Check sheet for the modelled part. Datum: model origin and axes. Units: mm. Face numbers are marked on the shaded views. Coordinates: 2 decimals unless noted, no trailing zeros. Loops run counter-clockwise (first coordinate to the right, second up) from the corner with the lowest first, then second, coordinate; pieces in that order, holes last.
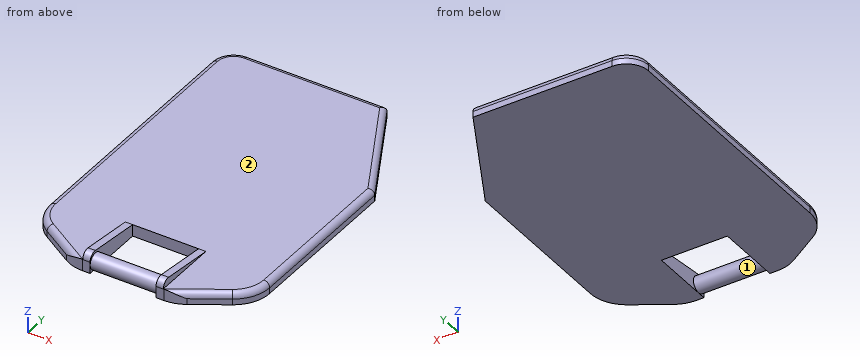
from build123d import *

# Parameters (mm, degrees)
F0_W          = 30
F0_H          = 45
F1_DEPTH      = 1.6
F2_SIZE2      = 8
F2_SIZE       = 5
F2_2_SIZE2    = 8
F2_2_SIZE     = 5
F3_R          = 3
F5_DEPTH      = 1.6
F6_W          = 11
F6_H          = 9
F7_DEPTH      = 2
F8_R          = 5
F10_DEPTH     = 1
F11_T1_DEPTH  = 6.6483183522
F13_DEPTH     = 1
F14_T1_DEPTH  = 6.6483183522
F16_T1_DEPTH  = 34.2287617925
F16_T3_DEPTH  = 24.2287617925
F16_T5_DEPTH  = 21
F16_T7_DEPTH  = 21
F16_T12_DEPTH = 8.6287617925
F16_T17_DEPTH = 8.6287617925
F16_T20_ANGLE = 57.9946167919
F16_T22_ANGLE = 90
F16_T24_ANGLE = 57.9946167919
F15_R         = 1.1066061355
F17_DEPTH     = 9


# Not quite as in the source:
# - a fillet or chamfer that OpenCascade refuses, or shapes differently, is made with other operations: its cross-section is extruded or revolved along the edge and cut away or added


with BuildPart() as f1:
    # F0 (on Top) → F1 (new body)
    with BuildSketch(Plane.XY):
        with Locations((-15, 22.5)):
            Rectangle(F0_W, F0_H)
    extrude(amount=F1_DEPTH)

    # F2
    f2_edges = [f1.edges().sort_by_distance(p)[0] for p in [
        (0, 0, 0.8),
    ]]
    f2_side = f1.faces().sort_by_distance((0, 22.5, 0.8))[0]
    chamfer(f2_edges, length=F2_SIZE, length2=F2_SIZE2, reference=f2_side)

    # F2#2
    f2_2_edges = [f1.edges().sort_by_distance(p)[0] for p in [
        (-30, 0, 0.8),
    ]]
    f2_2_side = f1.faces().sort_by_distance((-30, 22.5, 0.8))[0]
    chamfer(f2_2_edges, length=F2_2_SIZE, length2=F2_2_SIZE2, reference=f2_2_side)

    # F3
    f3_edges = [f1.edges().sort_by_distance(p)[0] for p in [
        (0, 45, 0.8),
        (-30, 45, 0.8),
    ]]
    fillet(f3_edges, radius=F3_R)

    # F4 (on face) → F5 (cut)
    with BuildSketch(Plane(origin=(0, 0, 0), x_dir=(1, 0, 0), z_dir=(0, 0, -1))):
        Polygon((0, -45), (0, -30), (-8, -45), align=None)
    extrude(amount=-F5_DEPTH, mode=Mode.SUBTRACT)

    # F6 (on face) → F7 (cut)
    with BuildSketch(Plane.XY.offset(1.6)):
        with Locations((-15, 4.5)):
            Rectangle(F6_W, F6_H)
    extrude(amount=-F7_DEPTH, mode=Mode.SUBTRACT)

    # F8
    f8_edges = [f1.edges().sort_by_distance(p)[0] for p in [
        (0, 5, 0.8),
        (-8, 0, 0.8),
        (-22, 0, 0.8),
        (-30, 5, 0.8),
    ]]
    fillet(f8_edges, radius=F8_R)

    # F9 (on face) → F10 (join)
    with BuildSketch(Plane(origin=(-9.5, 0, 0), x_dir=(0, -1, 0), z_dir=(-1, 0, 0))):
        Polygon((0, 2.7), (-9, 1.6), (-9, 0), (0, 0), align=None)
    extrude(amount=F10_DEPTH)

    # F11: fillet of radius 1 on 1 edges, made by hand

    # F11_s2 → F11_t1 (cut)
    with BuildSketch(Plane.YZ.offset(-13.3241591761)):
        with BuildLine():
            ThreePointArc((1.12131943, 2.5629498474), (0.3371725073, 2.3191084678), (0, 1.5703363296))
            Line((0, 1.5703363296), (0, 2.7))
            Line((0, 2.7), (1.12131943, 2.5629498474))
        make_face()
    extrude(amount=F11_T1_DEPTH, mode=Mode.SUBTRACT)

    # F12 (on face) → F13 (join)
    with BuildSketch(Plane.YZ.offset(-20.5)):
        Polygon((0, 2.7), (0, 0), (9, 0), (9, 1.6), align=None)
    extrude(amount=F13_DEPTH)

    # F14: fillet of radius 1 on 1 edges, made by hand

    # F14_s2 → F14_t1 (cut)
    with BuildSketch(Plane.YZ.offset(-23.3241591761)):
        with BuildLine():
            ThreePointArc((1.12131943, 2.5629498474), (0.3371725073, 2.3191084678), (0, 1.5703363296))
            Line((0, 1.5703363296), (0, 2.7))
            Line((0, 2.7), (1.12131943, 2.5629498474))
        make_face()
    extrude(amount=F14_T1_DEPTH, mode=Mode.SUBTRACT)

    # F16: fillet of radius 0.8 on 9 edges, made by hand

    # F16_s2 → F16_t1 (cut)
    with BuildSketch(Plane.XZ.offset(-42)):
        with BuildLine():
            ThreePointArc((-30, 0.8), (-29.7656854249, 1.3656854249), (-29.2, 1.6))
            Line((-29.2, 1.6), (-30, 1.6))
            Line((-30, 1.6), (-30, 0.8))
        make_face()
    extrude(amount=F16_T1_DEPTH, mode=Mode.SUBTRACT)

    # F16_s4 → F16_t3 (cut)
    with BuildSketch(Plane.XZ.offset(-32)):
        with BuildLine():
            ThreePointArc((0, 0.8), (-0.2343145751, 1.3656854249), (-0.8, 1.6))
            Line((-0.8, 1.6), (0, 1.6))
            Line((0, 1.6), (0, 0.8))
        make_face()
    extrude(amount=F16_T3_DEPTH, mode=Mode.SUBTRACT)

    # F16_s6 → F16_t5 (cut)
    with BuildSketch(Plane.YZ.offset(-27)):
        with BuildLine():
            ThreePointArc((45, 0.8), (44.7656854249, 1.3656854249), (44.2, 1.6))
            Line((44.2, 1.6), (45, 1.6))
            Line((45, 1.6), (45, 0.8))
        make_face()
    extrude(amount=F16_T5_DEPTH, mode=Mode.SUBTRACT)

    # F16_s8 → F16_t7 (cut)
    with BuildSketch(Plane(origin=(-11.5155709343, 21.5916955017, 0), x_dir=(0, 0, 1), z_dir=(-0.4705882353, 0.8823529412, 0))):
        with BuildLine():
            ThreePointArc((0.8, 14.1176470588), (1.3656854249, 13.8833324838), (1.6, 13.3176470588))
            Line((1.6, 13.3176470588), (1.6, 14.1176470588))
            Line((1.6, 14.1176470588), (0.8, 14.1176470588))
        make_face()
    extrude(amount=F16_T7_DEPTH, mode=Mode.SUBTRACT)


with BuildPart() as f16_tool10:
    # F16_s11 → F16_t12 (new body)
    with BuildSketch(Plane(origin=(-21.4702194191, 13.4188871369, 0), x_dir=(0, 0, 1), z_dir=(0.847998304, -0.52999894, 0))):
        with BuildLine():
            ThreePointArc((0.8, 11.6599766801), (1.3656854249, 11.425662105), (1.6, 10.8599766801))
            Line((1.6, 10.8599766801), (1.6, 11.6599766801))
            Line((1.6, 11.6599766801), (0.8, 11.6599766801))
        make_face()
    extrude(amount=F16_T12_DEPTH)

    split(bisect_by=Plane.YZ.offset(-20.5), keep=Keep.BOTTOM)


with BuildPart() as f1_1:
    add(f1.part)

    # F16_t9: cut F16_tool10
    add(f16_tool10.part, mode=Mode.SUBTRACT)


with BuildPart() as f16_tool15:
    # F16_s16 → F16_t17 (new body)
    with BuildSketch(Plane(origin=(-0.1028142887, -0.0642589305, 0), x_dir=(0, 0, 1), z_dir=(-0.847998304, -0.52999894, 0))):
        with BuildLine():
            ThreePointArc((0.8, 4.23999152), (1.3656854249, 4.4743060951), (1.6, 5.03999152))
            Line((1.6, 5.03999152), (1.6, 4.23999152))
            Line((1.6, 4.23999152), (0.8, 4.23999152))
        make_face()
    extrude(amount=F16_T17_DEPTH)

    split(bisect_by=Plane.YZ.offset(-9.5), keep=Keep.TOP)


with BuildPart() as f1_2:
    add(f1_1.part)

    # F16_t14: cut F16_tool15
    add(f16_tool15.part, mode=Mode.SUBTRACT)

    # F16_s19 → F16_t20 (revolve, cut)
    with BuildSketch(Plane.XZ.offset(-7.7712382075)):
        with BuildLine():
            ThreePointArc((0, 0.8), (-0.2343145751, 1.3656854249), (-0.8, 1.6))
            Line((-0.8, 1.6), (0, 1.6))
            Line((0, 1.6), (0, 0.8))
        make_face()
    revolve(axis=Axis((-5, 7.7712382075, 1.6), (0, 0, -1)), revolution_arc=F16_T20_ANGLE, mode=Mode.SUBTRACT)

    # F16_s21 → F16_t22 (revolve, cut)
    with BuildSketch(Plane.XZ.offset(-42)):
        with BuildLine():
            ThreePointArc((-30, 0.8), (-29.7656854249, 1.3656854249), (-29.2, 1.6))
            Line((-29.2, 1.6), (-30, 1.6))
            Line((-30, 1.6), (-30, 0.8))
        make_face()
    revolve(axis=Axis((-27, 42, 1.6), (0, 0, -1)), revolution_arc=F16_T22_ANGLE, mode=Mode.SUBTRACT)

    # F16_s23 → F16_t24 (revolve, cut)
    with BuildSketch(Plane(origin=(-21.4702194191, 13.4188871369, 0), x_dir=(0, 0, 1), z_dir=(0.847998304, -0.52999894, 0))):
        with BuildLine():
            ThreePointArc((0.8, 11.6599766801), (1.3656854249, 11.425662105), (1.6, 10.8599766801))
            Line((1.6, 10.8599766801), (1.6, 11.6599766801))
            Line((1.6, 11.6599766801), (0.8, 11.6599766801))
        make_face()
    revolve(axis=Axis((-25, 7.7712382075, 1.6), (0, 0, -1)), revolution_arc=F16_T24_ANGLE, mode=Mode.SUBTRACT)

    # F15 (on face) → F17 (join)
    with BuildSketch(Plane.YZ.offset(-19.5)):
        with Locations((1.125, 1.125)):
            Circle(F15_R)
    extrude(amount=F17_DEPTH)


solid = f1_2.part
(1) Scan lines: line 1 along X through (y, z) = (8, 0.2); line 2 along Z through (x, y) = (-18, 38); line 3 along X through (y, z) = (7, 1.2). Record each from-to range of solid material in increasing order.
(2) Draft check along Y on the marked faces 1 and 2. Enter one of: pulls with the +Y half, pulls with the -Y half, needs draft (parallel to the pull), parting line crosses it, or undercut.
(3) Gauge pin test, flat ends, axial feed: P1, Ø1.3, axis at y = 5, z = 1.5, coming from the -X side; P2, Ø6, axis at x = -10.5, y = 6.5, coming from the +Z side; P3, Ø1, axis at y = 10.5, z = 1.5, coming from the +X side. Record the tip position at first contact, or that the pin passes through.
(4) Section check A-A, the plane x = -20. Enter the section's corners in (y, z), plus the area to 3 significant figures.
(5) Section check B-B, the plane y = 29. Enter the section's corners in (x, z), plus the area to 3 significant figures.
Determined:
1. line 1: x = -30 to -19.5, -10.5 to 0
1. line 2: z = 0 to 1.6
1. line 3: x = -29.83 to -19.5, -10.5 to -0.17
2. face 1: undercut
2. face 2: needs draft
3. P1: stops at x = -29.4
3. P2: stops at z = 2.27
3. P3: stops at x = -0.03
4. outline: (0, 0) - (45, 0) - (45, 0.8) arc R0.8 ccw to (44.2, 1.6) - (9, 1.6) - (1.12, 2.56) arc R1 ccw to (0, 1.57) - close
4. area: 76.5 mm2
5. outline: (-30, 0) - (0, 0) - (0, 0.8) arc R0.8 ccw to (-0.8, 1.6) - (-29.2, 1.6) arc R0.8 ccw to (-30, 0.8) - close
5. area: 47.7 mm2
